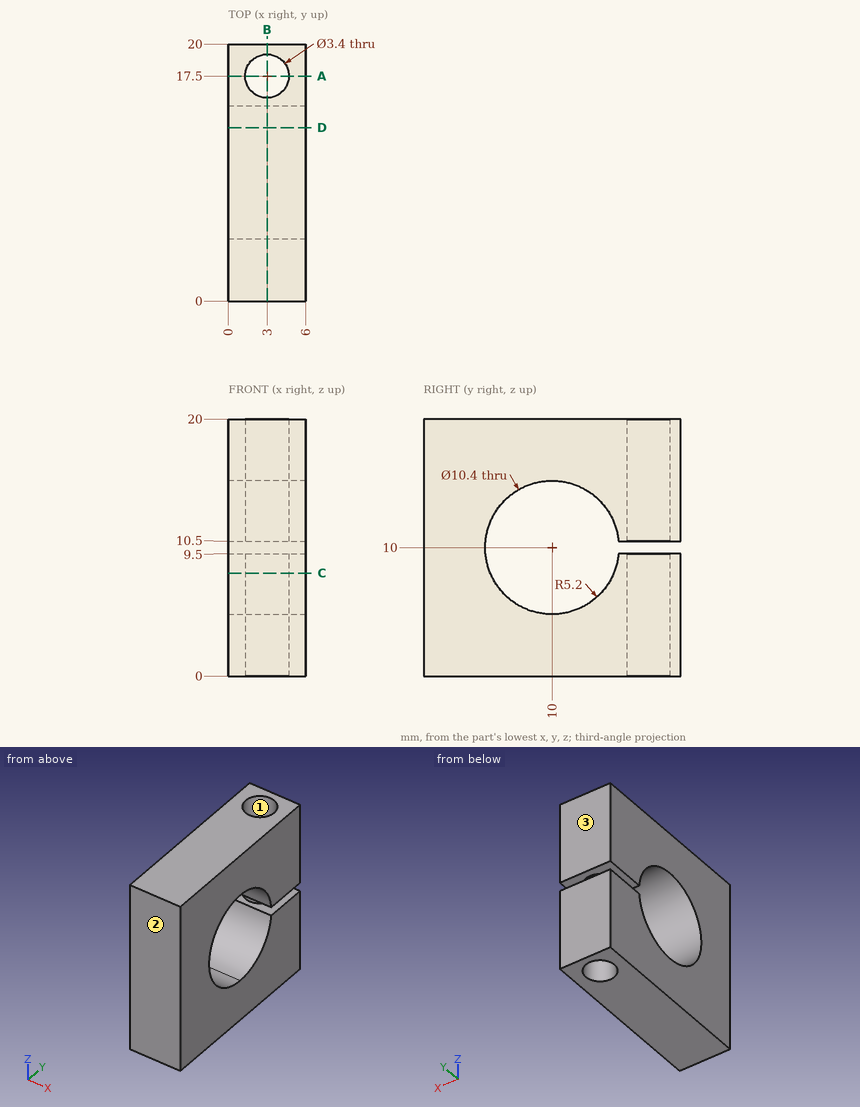
Geometry check sheet. Reference: drawing and pictorial views, mm from the part's lowest x, y, z. Give positions to 0.01 mm unless a question says otherwise; leave off trailing zeros. Order: outer loops, then holes, each group sorted by start corner. A loop starts at its lowest first (then second) coordinate and runs counter-clockwise, first axis right, second up. Notation, with made-up numbers: M 9.25,45.25 L 41.25,45.25 A22 ccw 41.25,68.25 Z; hole C -13.75,82 d3. An arc over 180 degrees is marked long. Answer as a JSON object with one key per item and string values. Group by question number.
1) Cross-section at B-B (x = 3). Enter the section's corners in (y, z), then the cut area to 3 significant figures.
2) Mould release check, pull along Y, two halves, no side actions. Record for the marked faces 1, 2 and 3: released by +Y, released by -Y, zero draft, split by the parting line, or undercut.
3) Cross-section at C-C (z = 8). Enter the section's corners in (x, y), then the cut area to 3 significant figures.
4) Cross-section at D-D (y = 13.5). Enter the section's corners in (x, z), then the cut area to 3 significant figures.
5) Scan lines: line 1 along Z through (x, y) = (4.75, 10); line 2 along Y through (x, z) = (3.6, 11.75); line 3 along X through (y, z) = (17.5, 7.25). Record each from-to range of solid material in increasing order. Write a range as [from, to].
6) Cross-section at A-A (y = 17.5). Enter the section's corners in (x, z).
Result sheet:
{
 "1": {"outline": "M 0,0 L 15.8,0 L 15.8,9.5 L 15.18,9.5 A5.2 cw long 15.18,10.5 L 15.8,10.5 L 15.8,20 L 0,20 Z; M 19.2,0 L 20,0 L 20,9.5 L 19.2,9.5 Z; M 19.2,10.5 L 20,10.5 L 20,20 L 19.2,20 Z", "area": "246 mm2"},
 "2": {"face 1": "undercut", "face 2": "released by -Y", "face 3": "released by +Y"},
 "3": {"outline": "M 0,0 L 6,0 L 6,5.2 L 0,5.2 Z; M 0,14.8 L 6,14.8 L 6,20 L 0,20 Z; hole C 3,17.5 d3.4", "area": "53.3 mm2"},
 "4": {"outline": "M 0,0 L 6,0 L 6,6.15 L 0,6.15 Z; M 0,13.85 L 6,13.85 L 6,20 L 0,20 Z", "area": "73.9 mm2"},
 "5": {"line 1": "z = [0, 4.8], [15.2, 20]", "line 2": "y = [0, 5.1], [14.9, 15.91], [19.09, 20]", "line 3": "x = [0, 1.3], [4.7, 6]"},
 "6": {"outline": "M 0,0 L 1.3,0 L 1.3,9.5 L 0,9.5 Z; M 0,10.5 L 1.3,10.5 L 1.3,20 L 0,20 Z; M 4.7,0 L 6,0 L 6,9.5 L 4.7,9.5 Z; M 4.7,10.5 L 6,10.5 L 6,20 L 4.7,20 Z"}
}
